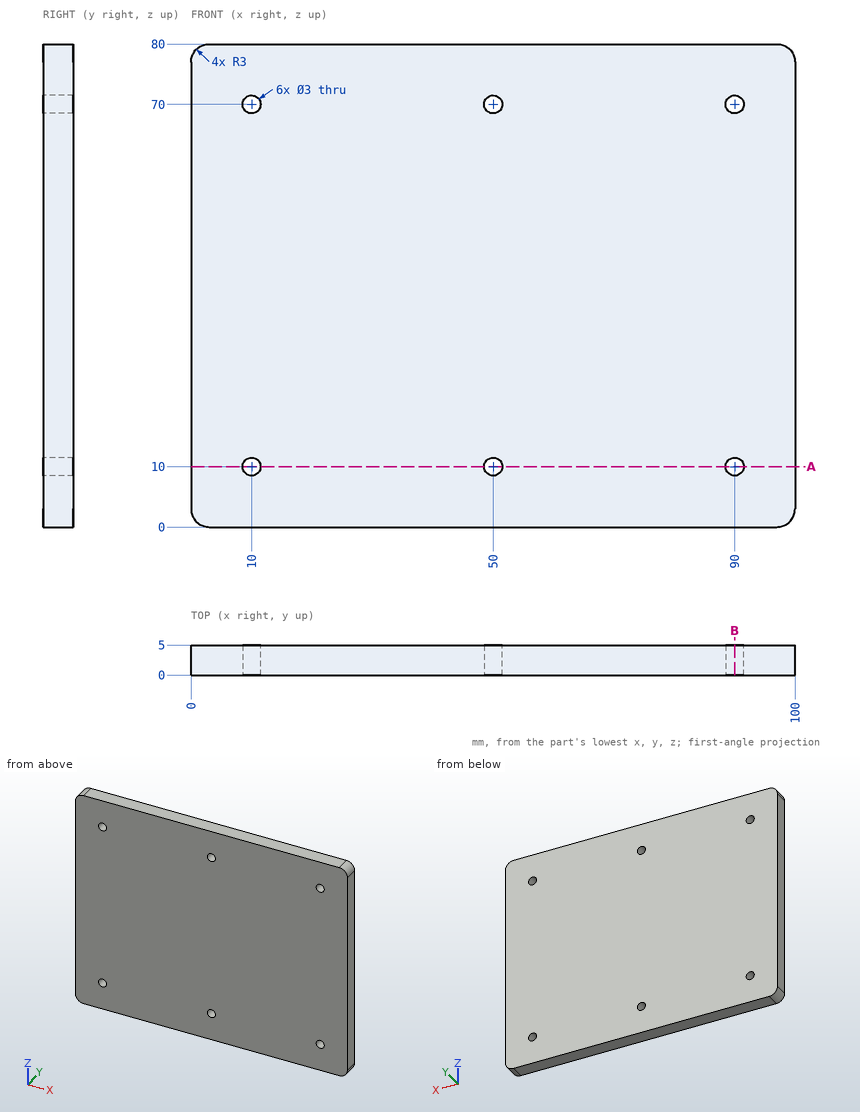
Verification items for this drawing (mm, ordinates from the low corner). Coordinates: 2 decimals unless noted, no trailing zeros. Loops run counter-clockwise (first coordinate to the right, second up) from the corner with the lowest first, then second, coordinate; pieces in that order, holes last. Notation, with made-up numbers: (-38.5, 62.25) - (-24.5, 62.25) arc R20 ccw to (-24.5, 90.25) - close; hole circle Ø4 at (46.25, 24). An arc over 180 degrees is marked (long way). Answer as a JSON object with one key per item and string values.
(1) Scan lines: line 1 along Z through (x, y) = (10, 3.7); line 2 along X through (y, z) = (2.1, 70); line 3 along Z through (x, y) = (91, 1.4). Record each from-to range of solid material in increasing order.
Response:
{"line 1": "z = 0 to 8.5, 11.5 to 68.5, 71.5 to 80", "line 2": "x = 0 to 8.5, 11.5 to 48.5, 51.5 to 88.5, 91.5 to 100", "line 3": "z = 0 to 8.88, 11.12 to 68.88, 71.12 to 80"}
(2) Cross-section at B-B, the plane x = 90. Record the boundary of the cut face in (y, z).
Response:
{"outline": "(0, 0) - (5, 0) - (5, 8.5) - (0, 8.5) - close; (0, 11.5) - (5, 11.5) - (5, 68.5) - (0, 68.5) - close; (0, 71.5) - (5, 71.5) - (5, 80) - (0, 80) - close"}
(3) Cross-section at A-A, the plane z = 10. Record the boundary of the cut face in (x, y), then the cut area to 3 significant figures.
Response:
{"outline": "(0, 0) - (8.5, 0) - (8.5, 5) - (0, 5) - close; (11.5, 0) - (48.5, 0) - (48.5, 5) - (11.5, 5) - close; (51.5, 0) - (88.5, 0) - (88.5, 5) - (51.5, 5) - close; (91.5, 0) - (100, 0) - (100, 5) - (91.5, 5) - close", "area": "455 mm²"}
